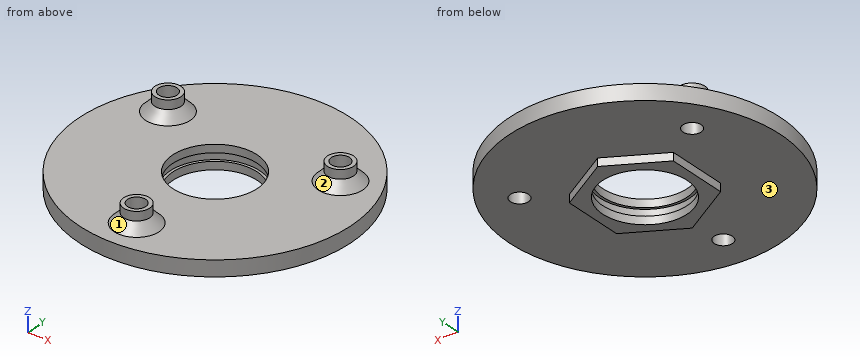
Autodesk Inventor part; units mm, degrees
ref_plane "Work Plane2" through (0, 0, -1.5) normal (0, 0, 1) x (1, 0, 0)
ref_plane "YZ Plane" through (0, 0, 0) normal (1, 0, 0) x (0, 1, 0)
ref_plane "XZ Plane" through (0, 0, 0) normal (0, 1, 0) x (-1, 0, 0)
sketch "Sketch3" plane through (0, 0, 0) normal (0, 0, 1) x (1, 0, 0)
  circle A0 centre (0, 0) radius 26
  dimension "d11" = 52
sketch "Sketch4" plane through (0, 0, 0) normal (0, 0, 1) x (1, 0, 0)
  circle A0 centre (0, -19.155) radius 1.75
  circle A1 centre (0, -19.155) radius 2.5
  circle A2 centre (0, -19.155) radius 5
  circle A3 centre (16.5887, 9.5775) radius 1.75
  circle A4 centre (16.5887, 9.5775) radius 2.5
  circle A5 centre (16.5887, 9.5775) radius 5
  circle A6 centre (-16.5887, 9.5775) radius 1.75
  circle A7 centre (-16.5887, 9.5775) radius 2.5
  circle A8 centre (-16.5887, 9.5775) radius 5
  point P0 (0, 0)
  dimension "d12" = 3.5
  dimension "d13" = 5
  dimension "d14" = 19.155
  dimension "d15" = 10
  dimension "d18" = 360
extrude "Extrusion1" add sketch "Sketch3" against normal blind 3
extrude "Extrusion3" add sketch "Sketch4" along normal blind 3.5 contours A1 | A4 | A7
chamfer "Chamfer1" distance 1.8 angle 45 3 edges at (14.0887, 9.5775, 0) (-19.0887, 9.5775, 0) (-2.5, -19.155, 0)
sketch "Sketch5" plane through (0, 0, -3) normal (0, 0, -1) x (-1, 0, 0)
  circle A0 centre (0, 0) radius 8.1
  dimension "d30" = 16.2
extrude "Extrusion4" cut sketch "Sketch5" against normal up to next
extrude "Extrusion8" cut sketch "Sketch4" against normal through all contours A0 | A3 | A6
sketch "Sketch8" plane through (0, 0, -3) normal (0, 0, -1) x (-1, 0, 0)
  circle A0 centre (0, 0) radius 8.1
  circle A1 centre (0, 0) radius 8.1
  line L0 (10, 5.7735) -> (10, -5.7735)
  line L1 (10, -5.7735) -> (0, -11.547)
  line L2 (0, -11.547) -> (-10, -5.7735)
  line L3 (-10, -5.7735) -> (-10, 5.7735)
  line L4 (-10, 5.7735) -> (0, 11.547)
  line L5 (0, 11.547) -> (10, 5.7735)
  dimension "d46" = 10
  dimension "d53" = 16.2
extrude "Extrusion10" add sketch "Sketch8" along normal blind 1.5
sketch "Sketch9" plane through (0, 0, 0) normal (0, 0, 1) x (1, 0, 0)
  circle A0 centre (0, 0) radius 8.0468
  circle A1 centre (0, 0) radius 8.6
  dimension "d49" = 17.2
ref_plane "Work Plane2" through (0, 0, -1.5) normal (0, 0, 1) x (1, 0, 0)
extrude "Extrusion11" cut sketch "Sketch9" against normal blind 1.5 from surface at -1.5
properties part number "Planet Carrier"
CAD build for the part. Positions are in the model's coordinates, mm. Face numbers are marked on the shaded views. Give positions to 0.01 mm unless a question says otherwise; leave off trailing zeros. Write each loop counter-clockwise with the first axis right and the second up, starting at its lowest first coordinate (ties: lowest second). Pieces come first, ordered by that corner, then holes. Notation, with made-up numbers: M 82.5,36 L 128.5,36 A23 cw 128.5,58 Z; hole C 22.5,45.5 d1. An arc over 180 degrees is marked long. Return JSON: item names as keys, results as strings. Group by question number.
(1) Band-saw the part on C-C (x = 21.5). Give the cut face in (y, z).
(2) Band-saw the part on D-D (y = 22). Give the cut face in (x, z).
(3) Drill centre lines: L1, parallel to Y at x = 0, z = -0.6 (3 decimals); L2, parallel to Y at x = 0, z = -2.6 (3 decimals); L3, parallel to Z at x = 6.5, y = -12. Where is each one in solid material? Low to high. Write a range as [from, to].
(4) Band-saw the part on A-A (z = 2.5). State how many separate pieces and enclosed holes the cut face has, and give its area (3 significant figures).
(5) Flat gauge pins, fed straight in: pin 1 Ø14 at (x, y) = (-2, 2.5) entering from +Z; pin 2 Ø1 at (y, z) = (6.5, 2.5) entering from +X; pin 3 Ø1.5 at (x, y) = (-9, 18.5) entering from -Z; pin 4 Ø3 at (y, z) = (4, 0) entering from +X. Where does each tip first touch, or does it go through?
(6) Mould opens along X. For the marked faces 1, 2 and 3 say: pulls with the +X half, pulls with the -X half, needs draft (parallel to the pull), parting line crosses it, or undercut.
(7) Band-saw the part on B-B (y = 0). Give the cut face in (x, z), and give its area (3 significant figures).
Entries:
{
 "1": {"outline": "M -14.62,-3 L 14.62,-3 L 14.62,0 L -14.62,0 Z"},
 "2": {"outline": "M -13.86,-3 L 13.86,-3 L 13.86,0 L -13.86,0 Z"},
 "3": {"L1": "y = [-26, -20.905], [-17.405, -8.1], [8.1, 26]", "L2": "y = [-26, -20.905], [-17.405, -8.6], [8.6, 26]", "L3": "z = [-3, 0]"},
 "4": {"separate pieces": "3", "enclosed holes": "3", "area": "30.0 mm^2"},
 "5": {"pin 1": "stops at z = 0", "pin 2": "passes through", "pin 3": "stops at z = -3", "pin 4": "stops at x = 25.88"},
 "6": {"face 1": "parting line crosses it", "face 2": "undercut", "face 3": "needs draft"},
 "7": {"outline": "M -26,-3 L -10,-3 L -10,-4.5 L -8.1,-4.5 L -8.1,-3 L -8.6,-3 L -8.6,-1.5 L -8.1,-1.5 L -8.1,0 L -26,0 Z; M 8.1,-4.5 L 10,-4.5 L 10,-3 L 26,-3 L 26,0 L 8.1,0 L 8.1,-1.5 L 8.6,-1.5 L 8.6,-3 L 8.1,-3 Z", "area": "112 mm^2"}
}
